from build123d import *

# Parameters (mm, degrees)
CYLINDER019_R             = 1
CYLINDER019_DEPTH         = 5
CYLINDER018_R             = 2.5
CYLINDER018_DEPTH         = 8
CYLINDER017_R             = 5
CYLINDER017_DEPTH         = 6
BOX002_W                  = 18
BOX002_H                  = 5
BOX002_DEPTH              = 2
CUT002002_PITCH_ANGLE     = 90
CUT002002_PLACEMENT_ANGLE = -90


with BuildPart() as cylinder019:
    # Cylinder019 → Cylinder019 (new body)
    with BuildSketch(Plane(origin=(0, 0, 3), x_dir=(0, 0, 1), z_dir=(-1, 0, 0))):
        Circle(CYLINDER019_R)
    extrude(amount=CYLINDER019_DEPTH)


with BuildPart() as fusion009:
    # Cylinder018 → Cylinder018 (new body)
    with BuildSketch(Plane.XY):
        Circle(CYLINDER018_R)
    extrude(amount=CYLINDER018_DEPTH)

    # Fusion009: union Cylinder019
    add(cylinder019.part)


with BuildPart() as cylinder017:
    # Cylinder017 → Cylinder017 (new body)
    with BuildSketch(Plane.XY):
        Circle(CYLINDER017_R)
    extrude(amount=CYLINDER017_DEPTH)


with BuildPart() as obj1:
    # Box002 → Box002 (new body)
    with BuildSketch(Plane(origin=(0, -2.5, 2), x_dir=(1, 0, 0), z_dir=(0, 0, 1))):
        with Locations((9, 2.5)):
            Rectangle(BOX002_W, BOX002_H)
    extrude(amount=BOX002_DEPTH)

    # Fusion008: union Cylinder017
    add(cylinder017.part)

    # Cut002002: cut Fusion009
    add(fusion009.part, mode=Mode.SUBTRACT)


with BuildPart() as obj1_1:
    # Cut002002 pitch: moved
    add(obj1.part.rotate(Axis((0, 0, 0), (0, 1, 0)), CUT002002_PITCH_ANGLE))


with BuildPart() as obj1_2:
    # Cut002002 placement: moved
    add(obj1_1.part.moved(Location((0, 37, 0))).rotate(Axis((0, 37, 0), (0, 0, 1)), CUT002002_PLACEMENT_ANGLE))


solid = obj1_2.part
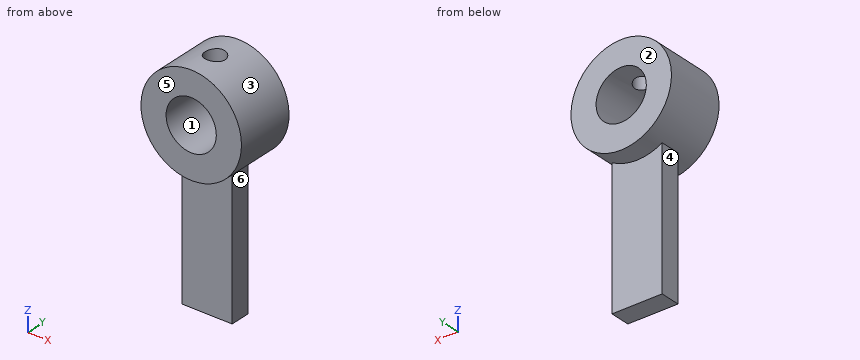
CAD build for the part. Positions are in the model's coordinates, mm. Face numbers are marked on the shaded views. A direction names the side the tool comes from. Coordinates: 2 decimals unless noted, no trailing zeros. Write each loop counter-clockwise with the first axis right and the second up, starting at its lowest first coordinate (ties: lowest second). Pieces come first, ordered by that corner, then holes. Notation, with made-up numbers: M -14.5,-6.5 L 0.5,-6.5 A18 ccw 0.5,24.5 Z; hole C 30,65.25 d1. An arc over 180 degrees is marked long. Answer as a JSON object with one key per item and string values. Group by question number.
1) Wall check: line 1 (X direction, y = 34, z = 0); line 2 (Y direction, x = 1.75, z = -12.75); line 3 (Y direction, x = 0.25, z = 3.75). Give the ranges that are in metal, low to high. Write a range as from..to.
2) Pin check, flat tips, straight feed: pin 1 Ø4 at (x, z) = (0, 0) entering from -Y; pin 2 Ø2.5 at (x, z) = (1, -9.5) entering from -Y; pin 3 Ø2.5 at (x, z) = (-1, -9.5) entering from +Y; pin 4 Ø1.6 at (y, z) = (34, -13.5) entering from -X. Stop position of each tip, or through.
3) Saw through at A-A (x = 0). Write the cut outline in (y, z), plus the area to 3 significant figures.
4) Saw through at C-C (y = 35.75). Write the cut outline in (x, z).
5) Tool access for the marked faces 4, 5 and 6: list every direction of +Z, -Z, +X, -X, +Y, -Y with a clear straight run to the whole face (end or side of a thin tool).
6) Saw through at D-D (x = 2). Write the cut outline in (y, z), plus the area to 3 significant figures.
7) Mould opens along X. For the marked faces 1, 2 and 3 say: +X half, -X half, draft (parallel to the pull), parting line (faces both ways), or undercut.
8) Saw through at B-B (z = 0). Write the cut outline in (x, y), plus the area to 3 significant figures.
Values follow:
{
 "1": {"line 1": "x = -5..-2.5, 2.5..5", "line 2": "y = 33..35", "line 3": "y = 31..33.03, 34.97..37"},
 "2": {"pin 1": "passes through", "pin 2": "stops at y = 33", "pin 3": "stops at y = 35", "pin 4": "stops at x = -2.5"},
 "3": {"outline": "M 31,-5 L 33,-5 L 33,-18 L 35,-18 L 35,-5 L 37,-5 L 37,-2.5 L 31,-2.5 Z; M 31,2.5 L 33,2.5 L 33,5 L 31,5 Z; M 35,2.5 L 37,2.5 L 37,5 L 35,5 Z", "area": "51.0 mm2"},
 "4": {"outline": "C 0,0 d10; hole C 0,0 d5"},
 "5": {"face 4": "-Z, -X, +Y, -Y", "face 5": "+Z, -Z, +X, -X, -Y", "face 6": "-Z, +X, +Y, -Y"},
 "6": {"outline": "M 31,-4.58 L 33,-4.58 L 33,-18 L 35,-18 L 35,-4.58 L 37,-4.58 L 37,-1.5 L 31,-1.5 Z; M 31,1.5 L 37,1.5 L 37,4.58 L 31,4.58 Z", "area": "63.8 mm2"},
 "7": {"face 1": "undercut", "face 2": "draft", "face 3": "parting line"},
 "8": {"outline": "M -5,31 L -2.5,31 L -2.5,37 L -5,37 Z; M 2.5,31 L 5,31 L 5,37 L 2.5,37 Z", "area": "30.0 mm2"}
}
